Autodesk Inventor part; units mm, degrees
ref_plane "YZ Plane" through (0, 0, 0) normal (1, 0, 0) x (0, 1, 0)
ref_plane "XZ Plane" through (0, 0, 0) normal (0, 1, 0) x (-1, 0, 0)
ref_plane "XY Plane" through (0, 0, 0) normal (0, 0, 1) x (1, 0, 0)
sketch "Sketch1" plane through (0, 0, 0) normal (0, 0, 1) x (1, 0, 0)
  line L0 (0, 0) -> (2.9, 0)
  line L1 (3, 0.1) -> (3, 10.5)
  line L2 (3, 10.5) -> (1.35, 10.5)
  line L3 (1.35, 10.5) -> (1.35, 13.5)
  line L4 (1.35, 13.5) -> (2.95, 13.5)
  line L5 (2.95, 13.5) -> (2.95, 19)
  line L6 (2.95, 19) -> (0.95, 19)
  line L7 (0.95, 19) -> (0.95, 0)
  line L8 (2.9, 0) -> (3, 0.1)
  line L9 (0.95, 0) -> (1.95, 0)
  line L10 (1.95, 0) -> (0.95, 0.5774)
  line L11 (0, 17.1506) -> (0, 0) construction
  dimension "d15" = 2.9
  dimension "d16" = 10.4
  dimension "d17" = 1.65
  dimension "d18" = 1.6
  dimension "d19" = 5.5
  dimension "d20" = 90
  dimension "d21" = 2
  dimension "d22" = 90
  dimension "d23" = 1
  dimension "d24" = 30
  dimension "d25" = 19
revolve "Revolution1" add sketch "Sketch1" angle 360 about axis through (0, 17.1506, 0) along (0, -1, 0) contours L10 L7 L6 L5 L4 L3 L2 L1 L8 L0
thread "Thread1"
chamfer "Chamfer1" distance 0.4 angle 45 2 edges at (-2.95, 19, 0) (-2.95, 13.5, 0)
chamfer "Chamfer2" distance 0.4 angle 45 1 edges at (-3, 10.5, 0)
properties part number "heatbreak ender 3s1" material "Titanium"
Could you check a few things on this model? Use its own coordinates, in mm. A direction names the side the tool comes from. Give positions to 0.01 mm unless a question says otherwise; leave off trailing zeros. Loops run counter-clockwise (first coordinate to the right, second up) from the corner with the lowest first, then second, coordinate; pieces in that order, holes last. Notation, with made-up numbers: M 85.25,44 L 110.25,44 A28 ccw 110.25,83 Z; hole C 44.25,41 d6. An arc over 180 degrees is marked long. Answer as a JSON object with one key per item and string values.
Q1. For P1, Ø1, axis at x = 0, z = 1, coming from the -Y side; P2, Ø1, axis at x = 2, y = 11.5, coming from the -Z side, each with a flat end and sliding along its axis, tell me the tip position at first contact or that it passes through.
Values found:
{"P1": "stops at y = 0.26", "P2": "passes through"}
Q2. If I drill on probe 1 along Z at (x, y) = (0, 8.75); probe 2 along Y at (x, z) = (1.9, 1.35); probe 3 along Z at (x, y) = (0, 12.75), over which ranges is the centre line in solid material (lowest first)? Write a range as [from, to].
Values found:
{"probe 1": "z = [-3, -0.95], [0.95, 3]", "probe 2": "y = [0, 10.5], [13.5, 19]", "probe 3": "z = [-1.35, -0.95], [0.95, 1.35]"}
Q3. For faces 5 (the cylindrical face through (-2.947, 16.283, -0.13)), 6 (the cylindrical face through (-0.29, 12.02, 1.32)), 7 (the flat face through (1, 0, -2)), which set-ups out of +Z, -Z, +X, -X, +Y, -Y let a thin tool reach every point of the face, with its end or its side?
Values found:
{"face 5": "+Y", "face 6": "none", "face 7": "+Z, -Z, +X, -X, -Y"}
Q4. If we mould it in two halves opening along Y, with no side actions, what happens to faces 1 (the flat face through (1.1, 13.5, -1.1)), 2 (the cylindrical face through (-0.95, 9.66, 0.04)), 3 (the flat face through (1.1, 19, 0)), 4 (the flat face through (1.1, 10.5, -1.1))? For each: pulls with the +Y half, pulls with the -Y half, needs draft (parallel to the pull), parting line crosses it, or undercut.
Values found:
{"face 1": "undercut", "face 2": "needs draft", "face 3": "pulls with the +Y half", "face 4": "undercut"}
Q5. Suppose I cut it at D-D, the plane y = 13. List the corners of the cut face in (x, z) for me, plus the area to 3 significant figures.
Values found:
{"outline": "C 0,0 d2.7; hole C 0,0 d1.9", "area": "2.89 mm²"}
Q6. Suppose I cut it at A-A, the plane x = 0. List the corners of the cut face in (y, z) for me.
Values found:
{"outline": "M 0,-2.9 L 0.1,-3 L 10.1,-3 L 10.5,-2.6 L 10.5,-1.35 L 13.5,-1.35 L 13.5,-2.55 L 13.9,-2.95 L 18.6,-2.95 L 19,-2.55 L 19,-0.95 L 0.58,-0.95 L 0,-1.95 Z; M 0,1.95 L 0.58,0.95 L 19,0.95 L 19,2.55 L 18.6,2.95 L 13.9,2.95 L 13.5,2.55 L 13.5,1.35 L 10.5,1.35 L 10.5,2.6 L 10.1,3 L 0.1,3 L 0,2.9 Z"}
Q7. Suppose I cut it at B-B, the plane z = 0. List the corners of the cut face in (x, y) for me.
Values found:
{"outline": "M -3,0.1 L -2.9,0 L -1.95,0 L -0.95,0.58 L -0.95,19 L -2.55,19 L -2.95,18.6 L -2.95,13.9 L -2.55,13.5 L -1.35,13.5 L -1.35,10.5 L -2.6,10.5 L -3,10.1 Z; M 0.95,0.58 L 1.95,0 L 2.9,0 L 3,0.1 L 3,10.1 L 2.6,10.5 L 1.35,10.5 L 1.35,13.5 L 2.55,13.5 L 2.95,13.9 L 2.95,18.6 L 2.55,19 L 0.95,19 Z"}
Q8. Suppose I cut it at C-C, the plane y = 2.5. List the corners of the cut face in (x, z) for me, plus the area to 3 significant figures.
Values found:
{"outline": "C 0,0 d6; hole C 0,0 d1.9", "area": "25.4 mm²"}
